Input: part model. Units: mm. Frame: model coordinates. A direction names the side the tool comes from. Give positions to 0.01 mm unless a question says otherwise; leave off trailing zeros. Write each loop counter-clockwise with the first axis right and the second up, starting at its lowest first coordinate (ties: lowest second). Pieces come first, ordered by that corner, then holes. Notation, with made-up numbers: (6.5, 17) - (18.5, 17) arc R25 cw to (18.5, 37) - close; hole circle Ø1 at (-22, 11). An arc over 180 degrees is marked (long way). Use a Markdown table: item, result. Add a question column.
1. Material intervals for probe 1 along X at (y, z) = (8.75, 7); probe 2 along Z at (x, y) = (-27, 1.2) (3 decimals); probe 3 along Z at (x, y) = (0.5, 4), sorted ascending.
2. Set-up query: faces 1 (the flat face through (17, 5.5, 8)), 2 (the flat face through (-25, 4, -22.5)), 3 (the flat face through (26, 3.5, 11)). Return all of +Z, -Z, +X, -X, +Y, -Y with unobstructed straight access to the full face (end or side cutting, diameter ignored); none if empty.
3. Section query A-A, the plane x = 0.09. Return loops of the section in (y, z), plus the area to 4 significant figures.
4. Mould query, pull axis Z, two halves, no side actions, for faces 4 (the flat face through (17, 5.5, -23)), 5 (the flat face through (-32, 4, 0)), 6 (the flat face through (0, 4, -29.5)). Classes: released by +Z, released by -Z, zero draft, split by the parting line, or undercut.
5. Section query B-B, the plane z = -14. Return loops of the section in (x, y), plus the area to 3 significant figures.
6. Section query C-C, the plane y = 2.25. Count the separate pieces of the cut face and the enclosed holes in it, plus the area to 3 significant figures.
7. Section query D-D, the plane x = -23.5. Return loops of the section in (y, z).
8. Pin query (flat end, axial travel): pin 1 (4.5 mm diameter, centred on x = -27, z = 12.5, fed in from -Y); pin 2 (3.5 mm diameter, centred on x = 25, y = 4, fed in from -Z); pin 3 (3.5 mm diameter, centred on x = -27, z = 12.5, fed in from +Y); pin 4 (1.7 mm diameter, centred on x = -27, z = -17.5, fed in from +Y). Return the tip coordinate at first contact, or that it passes through.
```python
from build123d import *

# Parameters (mm, degrees)
BOSS_EXTRUDE1_DEPTH = 9
SKETCH2_R           = 11.25
CUT_EXTRUDE1_DEPTH  = 9
SKETCH3_R           = 2.775
CUT_EXTRUDE2_DEPTH  = 3.5
SKETCH5_R           = 2.775
CUT_EXTRUDE4_DEPTH  = 3.5
SKETCH4_R           = 1.5
CUT_EXTRUDE3_DEPTH  = 6
SKETCH6_R           = 1.4
CUT_EXTRUDE5_DEPTH  = 6


with BuildPart() as part:
    # Sketch1 → Boss-Extrude1 (new body)
    with BuildSketch(Plane(origin=(0, 0, 0), x_dir=(1, 0, 0), z_dir=(0, 1, 0))):
        with BuildLine():
            Line((-15.5, 29.5), (15.5, 29.5))
            ThreePointArc((15.5, 29.5), (20.449747468, 27.449747468), (22.5, 22.5))
            Line((22.5, 22.5), (27, 22.5))
            ThreePointArc((27, 22.5), (30.535533906, 21.035533906), (32, 17.5))
            Line((32, 17.5), (32, -17.5))
            Line((32, -17.5), (-32, -17.5))
            Line((-32, -17.5), (-32, 17.5))
            ThreePointArc((-32, 17.5), (-30.535533906, 21.035533906), (-27, 22.5))
            Line((-27, 22.5), (-22.5, 22.5))
            ThreePointArc((-22.5, 22.5), (-20.449747468, 27.449747468), (-15.5, 29.5))
        make_face()
    extrude(amount=BOSS_EXTRUDE1_DEPTH)

    # Sketch2 → Cut-Extrude1 (cut)
    with BuildSketch(Plane(origin=(0, 9, 0), x_dir=(1, 0, 0), z_dir=(0, 1, 0))):
        with Locations((0.09, 8.5)):
            Circle(SKETCH2_R)
    extrude(amount=-CUT_EXTRUDE1_DEPTH, mode=Mode.SUBTRACT)

    # Sketch3 → Cut-Extrude2 (cut)
    with BuildSketch(Plane(origin=(0, 9, 0), x_dir=(1, 0, 0), z_dir=(0, 1, 0))):
        with Locations((-15.360283169, 23.950283169)):
            Circle(SKETCH3_R)
        with Locations((15.540283169, 23.950283169)):
            Circle(SKETCH3_R)
        with Locations((15.540283169, -6.950283169)):
            Circle(SKETCH3_R)
        with Locations((-15.360283169, -6.950283169)):
            Circle(SKETCH3_R)
    extrude(amount=-CUT_EXTRUDE2_DEPTH, mode=Mode.SUBTRACT)

    # Sketch5 → Cut-Extrude4 (cut)
    with BuildSketch(Plane(origin=(0, 0, 0), x_dir=(1, 0, 0), z_dir=(0, 1, 0))):
        with Locations((-27, 17.5)):
            Circle(SKETCH5_R)
        with Locations((27, 17.5)):
            Circle(SKETCH5_R)
        with Locations((27, -12.5)):
            Circle(SKETCH5_R)
        with Locations((-27, -12.5)):
            Circle(SKETCH5_R)
    extrude(amount=CUT_EXTRUDE4_DEPTH, mode=Mode.SUBTRACT)

    # Sketch4 → Cut-Extrude3 (cut)
    with BuildSketch(Plane(origin=(0, 5.5, 0), x_dir=(1, 0, 0), z_dir=(0, 1, 0))):
        with Locations((-15.360283169, 23.950283169)):
            Circle(SKETCH4_R)
        with Locations((15.540283169, 23.950283169)):
            Circle(SKETCH4_R)
        with Locations((15.540283169, -6.950283169)):
            Circle(SKETCH4_R)
        with Locations((-15.360283169, -6.950283169)):
            Circle(SKETCH4_R)
    extrude(amount=-CUT_EXTRUDE3_DEPTH, mode=Mode.SUBTRACT)

    # Sketch6 → Cut-Extrude5 (cut)
    with BuildSketch(Plane(origin=(0, 3.5, 0), x_dir=(-1, 0, 0), z_dir=(0, -1, 0))):
        with Locations((-27, -12.5)):
            Circle(SKETCH6_R)
        with Locations((-27, 17.5)):
            Circle(SKETCH6_R)
        with Locations((27, 17.5)):
            Circle(SKETCH6_R)
        with Locations((27, -12.5)):
            Circle(SKETCH6_R)
    extrude(amount=-CUT_EXTRUDE5_DEPTH, mode=Mode.SUBTRACT)


solid = part.part
```
Result sheet:
| question | item | result |
|---|---|---|
| 1 | probe 1 | x = -32 to -18.13, -12.59 to 12.77, 18.31 to 32 |
| 1 | probe 2 | z = -22.5 to -20.275, -14.725 to 9.725, 15.275 to 17.5 |
| 1 | probe 3 | z = -29.5 to -19.74, 2.74 to 17.5 |
| 2 | face 1 | +Y |
| 2 | face 2 | -Z, -X, +Y, -Y |
| 2 | face 3 | -Y |
| 3 | outline | (0, -29.5) - (9, -29.5) - (9, -19.75) - (0, -19.75) - close; (0, 2.75) - (9, 2.75) - (9, 17.5) - (0, 17.5) - close |
| 3 | area | 220.5 mm² |
| 4 | face 4 | undercut |
| 4 | face 5 | zero draft |
| 4 | face 6 | released by -Z |
| 5 | outline | (-32, 0) - (-9.72, 0) - (-9.72, 9) - (-32, 9) - close; (9.9, 0) - (32, 0) - (32, 9) - (9.9, 9) - close |
| 5 | area | 399 mm² |
| 6 | separate pieces | 1 |
| 6 | enclosed holes | 9 |
| 6 | area | 2,320 mm² |
| 7 | outline | (0, -22.5) - (9, -22.5) - (9, 17.5) - (0, 17.5) - close |
| 8 | pin 1 | stops at y = 3.5 |
| 8 | pin 2 | stops at z = -22.5 |
| 8 | pin 3 | stops at y = 9 |
| 8 | pin 4 | passes through |
